The model under review builds one solid part; all positions refer to its coordinate system, in mm. Give positions to 0.01 mm unless a question says otherwise; leave off trailing zeros. Loops run counter-clockwise (first coordinate to the right, second up) from the corner with the lowest first, then second, coordinate; pieces in that order, holes last. Notation, with made-up numbers: (44, -31) -> (87, -31) arc R7 cw to (87, -18) -> close; hole circle Ø11 at (-33.5, 22). An arc over 180 degrees is marked (long way). Write each question's results on one line, items separated by ' | '. Start each with the question number.
Q1. Mouldability with a two-part tool opening along Z and no side actions: class faces 1 (the face through (0, 1, 4)), 2 (the face through (0, 1, 2)), 3 (the face through (2, 3, -69)) as released by +Z, released by -Z, zero draft, split by the parting line, or undercut.
Q2. We need section C-C (y = 0.85). Write out the cut boundary in (x, z).
Q3. We need section B-B (x = 0). Write out the cut boundary in (y, z).
Q4. We need section A-A (z = -70). Write out the cut boundary in (x, y), plus the area to 3 significant figures.
Q5. Wall thickness on L1, parallel to Z at x = 0, y = 2.1; L2, parallel to Z at x = -1.25, y = 1; L3, parallel to X at y = 1.75, z = 0: over which ranges is each line inside the solid? List them lowest first. Write a range as [from, to].
Autodesk Inventor part; units mm, degrees
ref_plane "YZ Plane" through (0, 0, 0) normal (1, 0, 0) x (0, 1, 0)
ref_plane "XZ Plane" through (0, 0, 0) normal (0, 1, 0) x (-1, 0, 0)
ref_plane "XY Plane" through (0, 0, 0) normal (0, 0, 1) x (1, 0, 0)
sketch "Sketch1" plane through (0, 0, 0) normal (0, 1, 0) x (-1, 0, 0)
  circle A0 centre (0, 0) radius 2
  line L0 (0, 0) -> (0, -140)
  circle A1 centre (0, -140) radius 2
  circle A2 centre (0, -140) radius 4
  circle A3 centre (0, 0) radius 4
  line L1 (4, 0) -> (4, -140)
  line L2 (-4, 0) -> (-4, -140)
  line L3 (0, 0) -> (0, -70)
  circle A4 centre (0, -70) radius 2
  dimension "d0" = 4
  dimension "d1" = 140
  dimension "d2" = 4
  dimension "d3" = 8
  dimension "d4" = 8
  dimension "d7" = 70
  dimension "d8" = 4
extrude "Extrusion1" add sketch "Sketch1" along normal blind 3 contours A3 | A3 L1 A2 L0 A4 | L0 A4 A2 L2 A3 | A2
properties part number "tussenarmen_sturen"
Output:
1) face 1: released by +Z | face 2: undercut | face 3: zero draft
2) outline: (-4, -140) arc R4 ccw to (4, -140) -> (4, 0) arc R4 ccw to (-4, 0) -> close; hole circle Ø4 at (0, -140); hole circle Ø4 at (0, -70); hole circle Ø4 at (0, 0)
3) outline: (0, -144) -> (3, -144) -> (3, -142) -> (0, -142) -> close; (0, -138) -> (3, -138) -> (3, -72) -> (0, -72) -> close; (0, -68) -> (3, -68) -> (3, -2) -> (0, -2) -> close; (0, 2) -> (3, 2) -> (3, 4) -> (0, 4) -> close
4) outline: (-4, 0) -> (-2, 0) -> (-2, 3) -> (-4, 3) -> close; (2, 0) -> (4, 0) -> (4, 3) -> (2, 3) -> close | area: 12.0 mm2
5) L1: [-144, -142], [-138, -72], [-68, -2], [2, 4] | L2: [-143.8, -141.56], [-138.44, -71.56], [-68.44, -1.56], [1.56, 3.8] | L3: [-4, -2], [2, 4]
